from build123d import *

# Parameters (mm, degrees)
CUT_EXTRUDE1_DEPTH = 11.677078252


with BuildPart() as part:
    # Sketch1 → Revolve1 (revolve)
    with BuildSketch(Plane.XY):
        Polygon((0, 0), (-4, 0), (-4, 3.5), (0, 7), align=None)
    revolve(axis=Axis((0, 0, 0), (-1, 0, 0)))

    # Sketch2 → Cut-Extrude1 (cut, through all)
    with BuildSketch(Plane.ZY.offset(4)):
        Polygon((0, 3.290896534), (-2.85, 1.645448267), (-2.85, -1.645448267), (0, -3.290896534), (2.85, -1.645448267), (2.85, 1.645448267), align=None)
    extrude(amount=-CUT_EXTRUDE1_DEPTH, mode=Mode.SUBTRACT)


solid = part.part
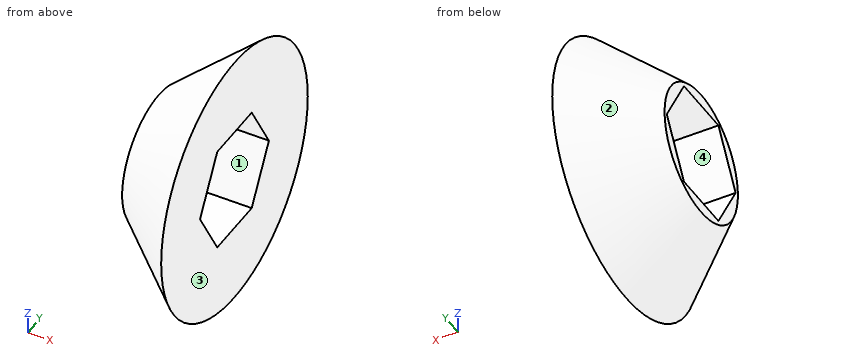
The listing builds one solid part. Answer for the finished solid, in the listing's coordinates (mm). Face numbers are marked on the shaded views. Give positions to 0.01 mm unless a question says otherwise; leave off trailing zeros. Write each loop counter-clockwise with the first axis right and the second up, starting at its lowest first coordinate (ties: lowest second). Pieces come first, ordered by that corner, then holes.
Item 1: Section C-C, the plane x = -0.75 is taken. Write down the section's boundary in (y, z), plus the area to 3 significant figures.
Item 2: Determine the mould class of the marked faces 1, 2, 3 and 4 for opening direction Y: released by +Y, released by -Y, zero draft, split by the parting line, or undercut.
Item 3: Flat-ended cylindrical pins translate along their axes: P1, Ø1, axis at x = -2, z = 4.5, coming from the +Y side; P2, Ø1, axis at x = -1, z = -5, coming from the +Y side. Find the tip coordinate at first contact, or state that the pin passes through.
Item 4: Section A-A, the plane y = 0 is taken. Write down the section's boundary in (x, z).
Item 5: Section B-B, the plane x = -2.4 is taken. Write down the section's boundary in (y, z), plus the area to 3 significant figures.
Item 6: Find the intervals of material crossed by line 1 along Y through (x, z) = (-2.75, -1.75); line 2 along Z through (x, y) = (-3.8, 1.25); line 3 along Y through (x, z) = (-3.55, 2), in increasing order.
Completed:
1. outline: circle Ø12.69 at (0, 0); hole (-3.29, 0) - (-1.65, -2.85) - (1.65, -2.85) - (3.29, 0) - (1.65, 2.85) - (-1.65, 2.85) - close
1. area: 98.3 mm2
2. face 1: undercut
2. face 2: split by the parting line
2. face 3: zero draft
2. face 4: undercut
3. P1: stops at y = 3.71
3. P2: stops at y = 4.45
4. outline: (-4, -3.5) - (0, -7) - (0, -2.85) - (-4, -2.85) - close; (-4, 2.85) - (0, 2.85) - (0, 7) - (-4, 3.5) - close
5. outline: circle Ø9.8 at (0, 0); hole (-3.29, 0) - (-1.65, -2.85) - (1.65, -2.85) - (3.29, 0) - (1.65, 2.85) - (-1.65, 2.85) - close
5. area: 47.3 mm2
6. line 1: y = -4.25 to -2.28, 2.28 to 4.25
6. line 2: z = -3.46 to -2.85, 2.85 to 3.46
6. line 3: y = -3.34 to -2.14, 2.14 to 3.34
